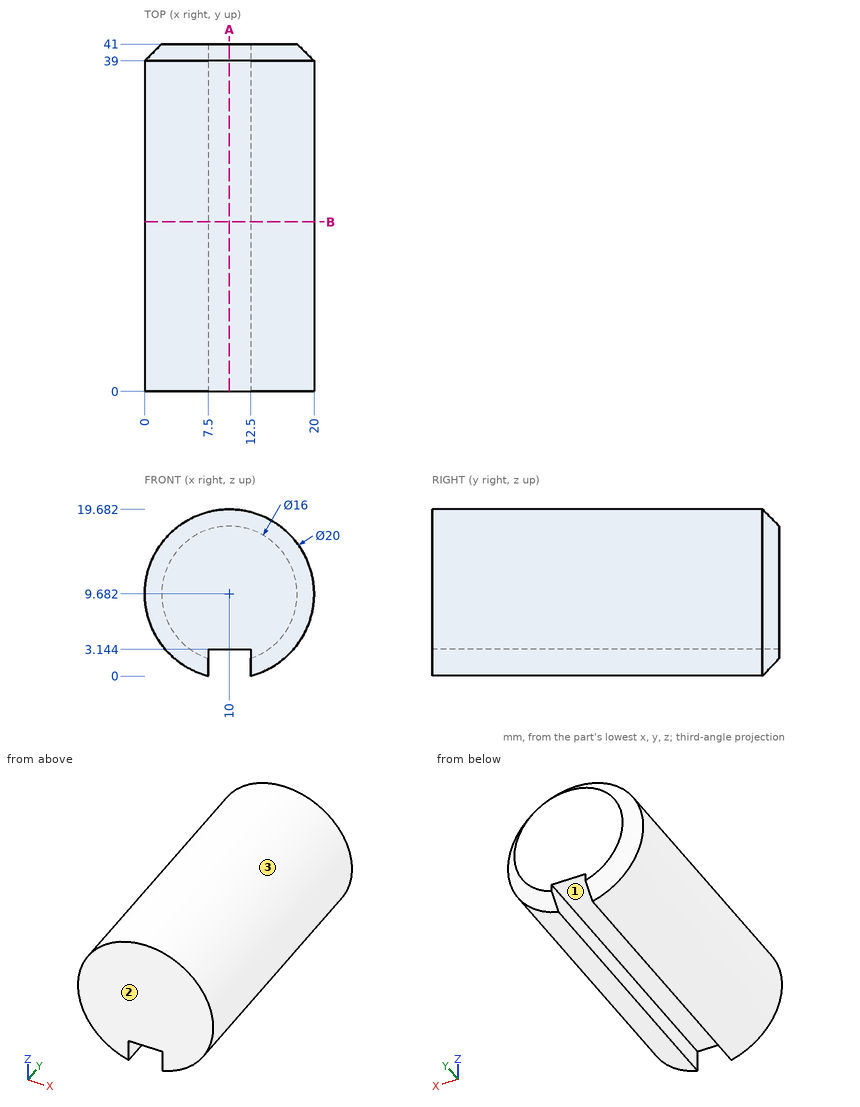
Geometry: see drawing. Coordinates: mm, zero at the bounding-box minimum. Give positions to 0.01 mm unless a question says otherwise; leave off trailing zeros. Write each loop counter-clockwise with the first axis right and the second up, starting at its lowest first coordinate (ties: lowest second). Pieces come first, ordered by that corner, then holes. Notation, with made-up numbers: M 47.5,62.25 L 52.5,62.25 A6 cw 52.5,71.25 Z; hole C 78,45 d11. An arc over 180 degrees is marked long. Answer in a Markdown table with one row per item. Add a question column.
(1) First-contact query: pin 1 (4 mm diameter, centred on x = 5, y = 11, fed in from -Z); pin 2 (2.5 mm diameter, centred on y = 23, z = 2.5, fed in from -X); pin 3 (1.5 mm diameter, centred on x = 16.5, y = 6.5, fed in from -Z). Flat tips, straight axial feed; report the tip coordinate or a pass-through.
(2) Mould query, pull axis X, two halves, no side actions, for the marked faces 1, 2 and 3. Classes: +X half, -X half, draft (parallel to the pull), parting line (faces both ways), or undercut.
(3) Section B-B on y = 20. Return loops of the section in (x, z) (1 decimal).
(4) Ray query, line 1 (X direction, y = 32.5, z = 9.5); line 2 (X direction, y = 25, z = 2.75) (1 decimal); line 3 (X direction, y = 14, z = 17) (1 decimal). Return the intervals inside material, ascending.
(5) Section A-A on x = 10. Return loops of the section in (y, z) (1 decimal), and give its area (3 significant figures).
Result set:
| question | item | result |
|---|---|---|
| 1 | pin 1 | stops at z = 0.14 |
| 1 | pin 2 | stops at x = 1.95 |
| 1 | pin 3 | stops at z = 1.5 |
| 2 | face 1 | undercut |
| 2 | face 2 | draft |
| 2 | face 3 | parting line |
| 3 | outline | M 7.5,0 L 7.5,3.1 L 12.5,3.1 L 12.5,0 A10 ccw long Z |
| 4 | line 1 | x = 0 to 20 |
| 4 | line 2 | x = 2.8 to 7.5, 12.5 to 17.2 |
| 4 | line 3 | x = 3.2 to 16.8 |
| 5 | outline | M 0,3.1 L 41,3.1 L 41,17.7 L 39,19.7 L 0,19.7 Z |
| 5 | area | 676 mm^2 |
